CAD build for the part. Positions are in the model's coordinates, mm. Face numbers are marked on the shaded views. A direction names the side the tool comes from. Give positions to 0.01 mm unless a question says otherwise; leave off trailing zeros. Order: outer loops, then holes, each group sorted by start corner. A loop starts at its lowest first (then second) coordinate and runs counter-clockwise, first axis right, second up. Notation, with made-up numbers: M -40,42 L 5,42 A5 cw 5,46 Z; hole C 29.5,39.25 d9. An arc over 180 degrees is marked long. Put each result on its own line as item: value. Start each with the question number.
1) Cut at B-B (y = 12.75). Write the cut outline in (x, z).
2) Cut at A-A (z = -40.5). Write the cut outline in (x, y), and give its area (4 significant figures).
3) Drill centre line: line 1 (X direction, y = 20.25, z = -39.5). Where is it in solid material? Low to high. Write a range as [from, to].
4) Tool access for the marked faces 1 and 2: list every direction of +Z, -Z, +X, -X, +Y, -Y with a clear straight run to the whole face (end or side of a thin tool).
5) Pin check, flat tips, straight feed: pin 1 (6 mm diameter, centred on x = -28.5, z = -54, fed in from -Y); pin 2 (1.5 mm diameter, centred on x = -70.5, z = -40.5, fed in from +Y); pin 3 (1 mm diameter, centred on y = 6, z = -33.5, fed in from -X). Stop position of each tip, or through.
```python
from build123d import *

# Parameters (mm, degrees)
SKETCH1_W      = 100
SKETCH1_H      = 35
EXTRUDE1_DEPTH = 24
SKETCH2_W      = 35
SKETCH2_H      = 5
EXTRUDE2_DEPTH = 5


with BuildPart() as part:
    # Sketch1 → Extrude1 (new body)
    with BuildSketch(Plane(origin=(0, 0, 0), x_dir=(1, 0, 0), z_dir=(0, 1, 0))):
        with Locations((-17.631525754, 40.747794601)):
            Rectangle(SKETCH1_W, SKETCH1_H)
    extrude(amount=EXTRUDE1_DEPTH)

    # Sketch2 → Extrude2 (add)
    with BuildSketch(Plane.ZY.offset(67.631525754)):
        with Locations((-40.747794601, 2.5)):
            Rectangle(SKETCH2_W, SKETCH2_H)
    extrude(amount=EXTRUDE2_DEPTH)


solid = part.part
```
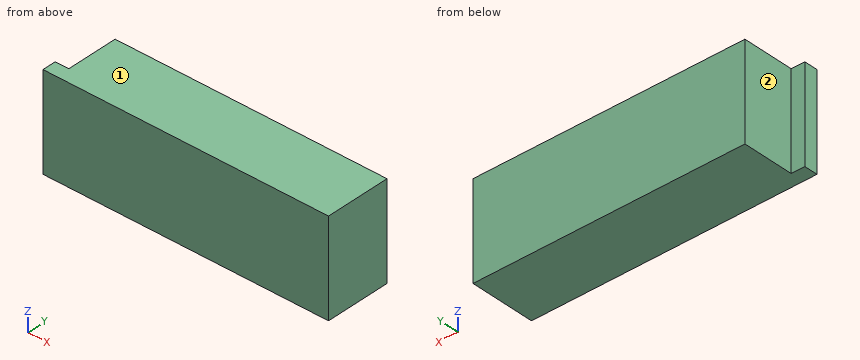
Solution:
1. outline: M -67.63,-58.25 L 32.37,-58.25 L 32.37,-23.25 L -67.63,-23.25 Z
2. outline: M -72.63,0 L 32.37,0 L 32.37,24 L -67.63,24 L -67.63,5 L -72.63,5 Z
2. area: 2,425 mm²
3. line 1: [-67.63, 32.37]
4. face 1: +Z, +X, -X, +Y, -Y
4. face 2: +Z, -Z, -X, +Y
5. pin 1: y = 0
5. pin 2: y = 5
5. pin 3: x = -67.63
